```python
from build123d import *

# Parameters (mm, degrees)
SKETCH_1_W      = 18.5
SKETCH_1_H      = 8.25
EXTRUDE_1_DEPTH = 15
SKETCH_2_R      = 3.75
EXTRUDE_2_DEPTH = 2
SKETCH_3_R      = 2.25
EXTRUDE_3_DEPTH = 2
SKETCH_4_R      = 1.9
EXTRUDE_4_DEPTH = 3.3
SKETCH_5_W      = 2
SKETCH_5_H      = 0.6
EXTRUDE_5_DEPTH = 1


with BuildPart() as part:
    # 草图1 → 凸台-拉伸1 (new body)
    with BuildSketch(Plane(origin=(0, 0, 0), x_dir=(1, 0, 0), z_dir=(0, 1, 0))):
        Rectangle(SKETCH_1_W, SKETCH_1_H)
    extrude(amount=EXTRUDE_1_DEPTH)

    # 草图2 → 凸台-拉伸2 (add)
    with BuildSketch(Plane(origin=(0, 15, 0), x_dir=(1, 0, 0), z_dir=(0, 1, 0))):
        with Locations((5.5, 0)):
            Circle(SKETCH_2_R)
    extrude(amount=EXTRUDE_2_DEPTH)

    # 草图3 → 凸台-拉伸3 (add)
    with BuildSketch(Plane(origin=(0, 15, 0), x_dir=(1, 0, 0), z_dir=(0, 1, 0))):
        with Locations((1.5, 0)):
            Circle(SKETCH_3_R)
    extrude(amount=EXTRUDE_3_DEPTH)

    # 草图4 → 凸台-拉伸4 (add)
    with BuildSketch(Plane(origin=(0, 17, 0), x_dir=(1, 0, 0), z_dir=(0, 1, 0))):
        with Locations((5.5, 0)):
            Circle(SKETCH_4_R)
    extrude(amount=EXTRUDE_4_DEPTH)

    # 草图5 → 凸台-拉伸5 (add)
    with BuildSketch(Plane(origin=(9.25, 0, 0), x_dir=(0, 0, -1), z_dir=(1, 0, 0))):
        with Locations((0, 3.8)):
            Rectangle(SKETCH_5_W, SKETCH_5_H)
    extrude(amount=EXTRUDE_5_DEPTH)


solid = part.part
```
CAD build for the part. Positions are in the model's coordinates, mm. A direction names the side the tool comes from. Coordinates: 2 decimals unless noted, no trailing zeros. Loops run counter-clockwise (first coordinate to the right, second up) from the corner with the lowest first, then second, coordinate; pieces in that order, holes last. Notation, with made-up numbers: (66.5, 38.25) - (75.5, 38.25) arc R23 ccw to (75.5, 47.25) - close; hole circle Ø10 at (32.25, -37). An arc over 180 degrees is marked (long way). Return JSON: item names as keys, results as strings.
1. Band-saw the part on B-B (x = 1.5). Give the cut face in (y, z) (3 decimals).
Result:
{"outline": "(0, -4.125) - (15, -4.125) - (15, -2.25) - (17, -2.25) - (17, 2.25) - (15, 2.25) - (15, 4.125) - (0, 4.125) - close"}
2. Band-saw the part on A-A (z = -3). Give the cut face in (x, y), and give its area (4 significant figures).
Result:
{"outline": "(-9.25, 0) - (9.25, 0) - (9.25, 15) - (7.75, 15) - (7.75, 17) - (3.25, 17) - (3.25, 15) - (-9.25, 15) - close", "area": "286.5 mm2"}
3. Mould opens along X. For faces 4 (the flat face through (10, 3.5, 0)), 5 (the cylindrical face through (-0.75, 15.99, -0.06)), 6 (the flat face through (-9.25, 7, 0)) say: released by +X, released by -X, zero draft, split by the parting line, or undercut.
Result:
{"face 4": "zero draft", "face 5": "undercut", "face 6": "released by -X"}
4. Probe L1, parallel to X at y = 14, z = -3.5; L2, parallel to Y at x = -4.25, z = -3; L3, parallel to Y at x = 7, z = 2. List the from-to ranges inside material, lowest first. Write a range as from..to.
Result:
{"L1": "x = -9.25..9.25", "L2": "y = 0..15", "L3": "y = 0..17"}
5. Drop a flat-ended pin along its axis: pin 1 (0.8 mm diameter, centred on x = 9.5, z = 0.5, fed in from +Y). Give the stop position or say it passes through.
Result:
{"pin 1": "stops at y = 17"}
6. Band-saw the part on C-C (y = 12.5). Give the cut face in (x, z) (3 decimals).
Result:
{"outline": "(-9.25, -4.125) - (9.25, -4.125) - (9.25, 4.125) - (-9.25, 4.125) - close"}
7. Band-saw the part on D-D (z = -1.5). Give the cut face in (x, y).
Result:
{"outline": "(-9.25, 0) - (9.25, 0) - (9.25, 15) - (8.94, 15) - (8.94, 17) - (6.67, 17) - (6.67, 20.3) - (4.33, 20.3) - (4.33, 17) - (-0.18, 17) - (-0.18, 15) - (-9.25, 15) - close"}
8. 3-axis set-ups, long thin cutter, end or side, ignore diameter. For faces 1 (the flat face through (10, 4.1, 0)), 2 (the flat face through (0, 0, 0)), 3 (the flat face through (3, 17, 0)): which of +Z, -Z, +X, -X, +Y, -Y reach the whole face in a straight line?
Result:
{"face 1": "+Z, -Z, +X, +Y", "face 2": "+Z, -Z, +X, -X, -Y", "face 3": "+Y"}
